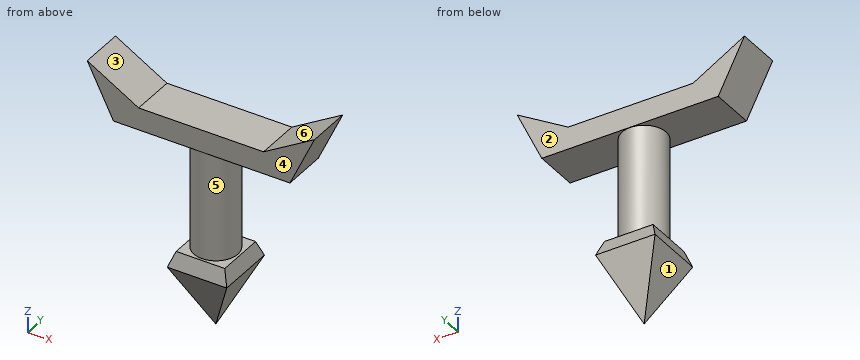
```python
from build123d import *

# Parameters (mm, degrees)
F0_W      = 50.8
F0_H      = 50.8
F1_FACE_W = 50.8
F1_FACE_H = 50.8
F2_DEPTH  = 12.7
F2_TAPER  = 20
F3_R      = 18.7690091821
F4_DEPTH  = 101.6
F6_DEPTH  = 19.05


# Not quite as in the source:
# - an extrude whose draft closes it to a point is written as a loft to that point


with BuildPart() as f1:
    # F0 (on Top) → F1 section 0
    with BuildSketch(Plane.XY, mode=Mode.PRIVATE) as f1_s0:
        Rectangle(F0_W, F0_H)
    loft([f1_s0.sketch, Vertex(0, 0, -54.4704757809)], ruled=True)

    # F1_face (on face) → F2 (join)
    with BuildSketch(Plane.XY):
        Rectangle(F1_FACE_W, F1_FACE_H)
    extrude(amount=F2_DEPTH, taper=F2_TAPER)

    # F3 (on face) → F4 (join)
    with BuildSketch(Plane.XY.offset(12.7)):
        Circle(F3_R)
    extrude(amount=F4_DEPTH)

    # F5 (on Front) → F6 (join, symmetric)
    with BuildSketch(Plane.XZ):
        Polygon((96.2837857294, 150.2247155843), (52.8015196323, 124.2486089468), (-53.8494151779, 124.2486089468), (-97.7485626936, 149.513810873), (-75.3541216254, 105.235889554), (75.3541216254, 105.235889554), align=None)
    extrude(amount=F6_DEPTH, both=True)


solid = f1.part
```
Source: CAD feature listing. Evaluate the final solid. Frame: model axes, mm. Face numbers are marked on the shaded views. A direction names the side the tool comes from. Give positions to 0.01 mm unless a question says otherwise; leave off trailing zeros. Write each loop counter-clockwise with the first axis right and the second up, starting at its lowest first coordinate (ties: lowest second). Pieces come first, ordered by that corner, then holes. Notation, with made-up numbers: (70.5, -40) - (86.5, -40) arc R15 cw to (86.5, -19) - close; hole circle Ø9 at (37.25, 20). An arc over 180 degrees is marked (long way). One line per item, written item: value. Start each with the question number.
Q1. Section query C-C, the plane x = -47. Return the cut outline in (y, z).
Q2. Section query D-D, the plane z = -36. Return the cut outline in (x, y).
Q3. Set-up query: the marked faces 1, 2 and 3. Return all of +Z, -Z, +X, -X, +Y, -Y with unobstructed straight access to the full face (end or side cutting, diameter ignored); none if empty.
Q4. Draft query along X for the marked faces 4, 5 and 6. Return one class per face: +X half, -X half, draft (parallel to the pull), parting line (faces both ways), or undercut.
Q5. First-contact query: pin 1 Ø2 at (y, z) = (-18.5, 116.5) entering from +X; pin 2 Ø19 at (x, y) = (15.5, 2) entering from +Z; pin 3 Ø22.5 at (x, z) = (-41, 125) entering from +Y. Flat tips, straight axial feed; report the tip coordinate or a pass-through.
Q6. Section query B-B, the plane y = -9. Return the cut outline in (x, z).
Q7. Section query A-A, the plane z = 132. Return the cut outline in (x, y).
Q8. Material intervals for probe 1 along Z at (x, y) = (-25.5, 13); probe 2 along X at (y, z) = (5, 129); probe 3 along Y at (x, z) = (16.5, 49), sorted ascending. Write a range as from..to.
Answer:
1. outline: (-19.05, 105.24) - (19.05, 105.24) - (19.05, 124.25) - (-19.05, 124.25) - close
2. outline: (-8.61, -8.61) - (8.61, -8.61) - (8.61, 8.61) - (-8.61, 8.61) - close
3. face 1: -Z, -X, +Y, -Y
3. face 2: +Z, +X, -X, +Y
3. face 3: +Z, +Y, -Y
4. face 4: draft
4. face 5: parting line
4. face 6: undercut
5. pin 1: stops at x = 81.06
5. pin 2: stops at z = 124.25
5. pin 3: stops at y = 19.05
6. outline: (-97.75, 149.51) - (-75.35, 105.24) - (-16.47, 105.24) - (-16.47, 12.7) - (-20.78, 12.7) - (-25.4, 0) - (-9, -35.17) - (9, -35.17) - (25.4, 0) - (20.78, 12.7) - (16.47, 12.7) - (16.47, 105.24) - (75.35, 105.24) - (96.28, 150.22) - (52.8, 124.25) - (-53.85, 124.25) - close
7. outline: (-88.89, -19.05) - (-67.32, -19.05) - (-67.32, 19.05) - (-88.89, 19.05) - close; (65.78, -19.05) - (87.81, -19.05) - (87.81, 19.05) - (65.78, 19.05) - close
8. probe 1: z = 105.24..124.25
8. probe 2: x = -87.37..-62.11, 60.76..86.41
8. probe 3: y = -8.95..8.95
